The drawing under review shows one solid part. Ordinate dimensions are in mm from its lowest x, y, z. Coordinates: 2 decimals unless noted, no trailing zeros. Write each loop counter-clockwise with the first axis right and the second up, starting at its lowest first coordinate (ties: lowest second). Pieces come first, ordered by that corner, then holes.
Q1. Add section A-A, the plane x = 26. Give the boundary of the cut face in (y, z).
Q2. Add section C-C, the plane y = 0.9. Give the boundary of the cut face in (x, z).
Q3. To check wall thickness, follow probe 1 along X at (y, z) = (0.85, 25); probe 2 along X at (y, z) = (1.35, 10); probe 3 along Z at (x, y) = (52.5, 0.75). State the ranges of each line that lie inside material, in increasing order.
Q4. Add section D-D, the plane z = 35.5. Give the boundary of the cut face in (x, y).
Q5. Add section B-B, the plane z = 10. Give the boundary of the cut face in (x, y).
Q6. Clearance check with flat-ended pins moving along their axes: pin 1 Ø2 at (x, z) = (19.5, 61) entering from -Y; pin 2 Ø3 at (x, z) = (55.5, 25) entering from +Y. State where each tip first meets the part, or that it passes through.
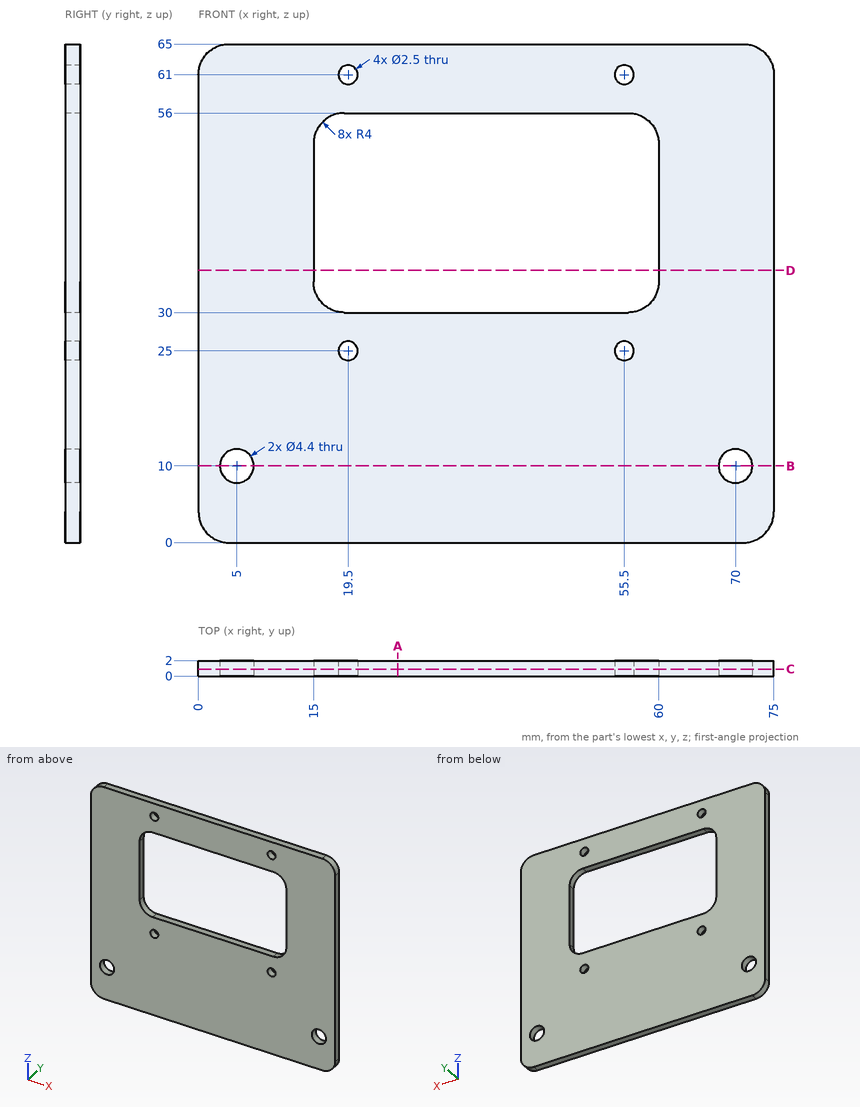
Here are the results:
1. outline: (0, 0) - (2, 0) - (2, 30) - (0, 30) - close; (0, 56) - (2, 56) - (2, 65) - (0, 65) - close
2. outline: (0, 4) arc R4 ccw to (4, 0) - (71, 0) arc R4 ccw to (75, 4) - (75, 61) arc R4 ccw to (71, 65) - (4, 65) arc R4 ccw to (0, 61) - close; hole circle Ø4.4 at (5, 10); hole (15, 34) arc R4 ccw to (19, 30) - (56, 30) arc R4 ccw to (60, 34) - (60, 52) arc R4 ccw to (56, 56) - (19, 56) arc R4 ccw to (15, 52) - close; hole circle Ø2.5 at (19.5, 25); hole circle Ø2.5 at (19.5, 61); hole circle Ø2.5 at (55.5, 25); hole circle Ø2.5 at (55.5, 61); hole circle Ø4.4 at (70, 10)
3. probe 1: x = 0 to 18.25, 20.75 to 54.25, 56.75 to 75
3. probe 2: x = 0 to 2.8, 7.2 to 67.8, 72.2 to 75
3. probe 3: z = 0 to 30, 56 to 65
4. outline: (0, 0) - (15, 0) - (15, 2) - (0, 2) - close; (60, 0) - (75, 0) - (75, 2) - (60, 2) - close
5. outline: (0, 0) - (2.8, 0) - (2.8, 2) - (0, 2) - close; (7.2, 0) - (67.8, 0) - (67.8, 2) - (7.2, 2) - close; (72.2, 0) - (75, 0) - (75, 2) - (72.2, 2) - close
6. pin 1: passes through
6. pin 2: stops at y = 2
